Here's how the part is built. I have some questions about the finished solid (model axes, mm). Face numbers are marked on the shaded views. Coordinates: 2 decimals unless noted, no trailing zeros. Write each loop counter-clockwise with the first axis right and the second up, starting at its lowest first coordinate (ties: lowest second). Pieces come first, ordered by that corner, then holes.
Item 1: I'm going to push flat-ended pins straight in: pin 1 Ø5.5 at (y, z) = (0, 0) entering from -X; pin 2 Ø1.3 at (x, y) = (-0.5, -0.5) entering from +Z; pin 3 Ø24 at (y, z) = (5, -18) entering from -X; pin 4 Ø4 at (x, y) = (-0.5, 22) entering from -Z. Where does each tip first touch, or does it pass through?
Item 2: If we section it at A-A (z = 7): Please give me the cut outline in (x, y), then the cut area to 3 significant figures.
Item 3: We'd pull the mould along Y, two halves only. Please class the marked faces 1, 2 and 3: +Y half, -Y half, draft (parallel to the pull), parting line (faces both ways), or undercut.
Item 4: If we section it at B-B (y = 23): Please give me the cut outline in (x, z).
Item 5: If we section it at D-D (z = -30.5): Please give me the cut outline in (x, y), then the cut area to 3 significant figures.
Item 6: If I drill on line 1 (Y direction, x = -3, z = 0) (3 decimals); line 2 (Z direction, x = -1, y = 21); line 3 (Y direction, x = -0.25, z = 10), over which ranges is the centre line in solid material (lowest first)?
Item 7: If we section it at C-C (x = -3.75): Please give me the cut outline in (y, z) (3 decimals).
from build123d import *

# Parameters (mm, degrees)
SKETCH3_W           = 5
SKETCH3_H           = 40
CUT_EXTRUDE1_DEPTH  = 5
CIRPATTERN1_COUNT   = 5
SKETCH8_R           = 2.75
BOSS_EXTRUDE1_DEPTH = 3
CUT_EXTRUDE2_REACH  = 10


with BuildPart() as part:
    # Sketch3 → Shape_Roue (revolve)
    with BuildSketch(Plane.XY):
        with Locations((0, 20)):
            Rectangle(SKETCH3_W, SKETCH3_H)
    revolve(axis=Axis((-2.5, 0, 0), (1, 0, 0)))

    # Sketch6 → Cut-Extrude1 (cut)
    with BuildSketch(Plane(origin=(2.5, 0, 0), x_dir=(0, 0, -1), z_dir=(1, 0, 0))):
        with BuildLine():
            Line((8.374067112, 8.374067112), (20.310096012, 20.310096012))
            ThreePointArc((20.310096012, 20.310096012), (23.415046761, 21.472099275), (26.330043569, 19.892933561))
            ThreePointArc((26.330043569, 19.892933561), (30.488024573, 12.628553268), (32.684580575, 4.551724138))
            ThreePointArc((32.684580575, 4.551724138), (31.740005351, 1.373871343), (28.722813233, 0))
            Line((28.722813233, 0), (11.842719282, 0))
            ThreePointArc((11.842719282, 0), (9.510338524, 0.750384638), (8.053049112, 2.72))
            ThreePointArc((8.053049112, 2.72), (7.852976026, 3.252809175), (7.617696081, 3.771035191))
            ThreePointArc((7.617696081, 3.771035191), (7.255426928, 6.194222796), (8.374067112, 8.374067112))
        make_face()
    cut_extrude1 = extrude(amount=-CUT_EXTRUDE1_DEPTH, mode=Mode.SUBTRACT)

    # CirPattern1: Cut-Extrude1 ×5 about axis
    cirpattern1_axis = Axis((0, 0, 0), (1, 0, 0))
    for i in range(1, CIRPATTERN1_COUNT):
        add(cut_extrude1.rotate(cirpattern1_axis, i * 360 / CIRPATTERN1_COUNT), mode=Mode.SUBTRACT)

    # Sketch8 → Boss-Extrude1 (add)
    with BuildSketch(Plane(origin=(-2.5, 0, 0), x_dir=(0, 0, -1), z_dir=(1, 0, 0))):
        Circle(SKETCH8_R)
    extrude(amount=-BOSS_EXTRUDE1_DEPTH)

    # Sketch7 → Cut-Extrude2 (cut, up to next)
    with BuildSketch(Plane(origin=(2.5, 0, 0), x_dir=(0, 0, -1), z_dir=(1, 0, 0)), mode=Mode.PRIVATE) as cut_extrude2_sk1:
        with BuildLine():
            Line((1.675, 1.307669683), (1.675, -1.307669683))
            ThreePointArc((1.675, -1.307669683), (-2.125, 0), (1.675, 1.307669683))
        make_face()
    cut_extrude2_tool1 = extrude(cut_extrude2_sk1.sketch, amount=-CUT_EXTRUDE2_REACH, mode=Mode.PRIVATE) & part.part
    add(cut_extrude2_tool1.solids().sort_by_distance((2.5, 0, 0.111388))[0], mode=Mode.SUBTRACT)


solid = part.part
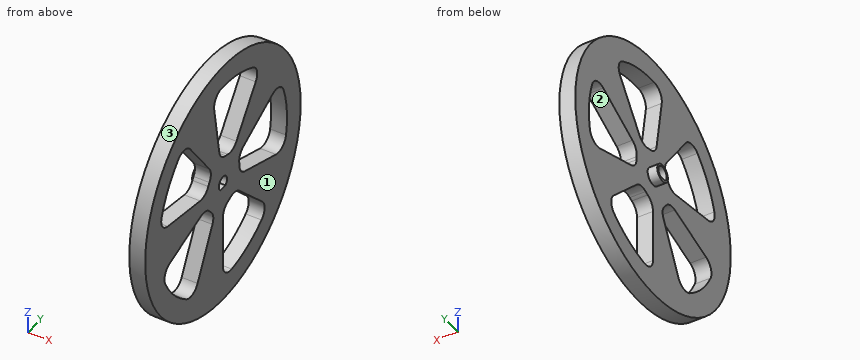
Answer list:
1. pin 1: stops at x = -5.5
1. pin 2: stops at z = 40
1. pin 3: stops at x = -2.5
1. pin 4: stops at z = -34.64
2. outline: (-2.5, -39.38) - (2.5, -39.38) - (2.5, -31.47) - (-2.5, -31.47) - close; (-2.5, -6.2) - (2.5, -6.2) - (2.5, 13.74) - (-2.5, 13.74) - close; (-2.5, 32.25) - (2.5, 32.25) - (2.5, 39.38) - (-2.5, 39.38) - close
2. area: 175 mm2
3. face 1: draft
3. face 2: undercut
3. face 3: parting line
4. outline: (-2.5, -32.73) - (2.5, -32.73) - (2.5, -7.47) - (-2.5, -7.47) - close; (-2.5, 11.72) - (2.5, 11.72) - (2.5, 32.73) - (-2.5, 32.73) - close
5. outline: (-2.5, -25.88) - (2.5, -25.88) - (2.5, 0.42) - (-2.5, 0.42) - close; (-2.5, 12.6) - (2.5, 12.6) - (2.5, 25.88) - (-2.5, 25.88) - close
5. area: 198 mm2
6. line 1: y = -2.75 to -2.125, 2.125 to 2.75
6. line 2: z = -34.04 to -25.04, -21.24 to -6.82, 10.7 to 34.04
6. line 3: y = -38.73 to -31.45, -7.27 to -1.16, 7.27 to 19.63, 31.45 to 38.73
7. outline: circle Ø5.5 at (0, 0); hole (-1.308, -1.675) - (1.308, -1.675) arc R2.125 ccw (long way) to start
